Can you work these out from the model? Positions are in its coordinate system, mm. Face numbers are marked on the shaded views. A direction names the side the tool comes from. Round coordinates to 2 decimals unless told otherwise and drop trailing zeros. Loops run counter-clockwise (first coordinate to the right, second up) from the corner with the lowest first, then second, coordinate; pieces in that order, holes last.
(1) If I drill on line 1 along Y through (x, z) = (9.25, 10.5); line 2 along Z through (x, y) = (6.75, 50); line 3 along Y through (x, z) = (8.75, 5), over which ranges is the centre line in solid material (lowest first)?
(2) I want a section at B-B on x = 0. Write out the boundary of the cut face in (y, z), plus the area to 3 significant figures.
(3) Which directions (+Z, -Z, +X, -X, +Y, -Y) give clear straight access to the entire face, cutting with the end or side of a thin tool? Please do the marked faces 1, 2 and 3.
(4) I want a section at A-A on z = 8.5. Write out the boundary of the cut face in (x, y), plus the area to 3 significant figures.
(5) I want a section at C-C on x = -10.5. Write out the boundary of the cut face in (y, z), plus the area to 3 significant figures.
(6) Will these pins go through, and if not, where does the flat tip stop? pin 1 Ø14.5 at (x, y) = (1.5, 42.5) entering from +Z; pin 2 Ø5.5 at (x, y) = (1, 46.5) entering from -Z; pin 3 Ø6 at (y, z) = (-43, 12.5) entering from +X; pin 4 Ø9 at (y, z) = (53.5, 11) entering from -X.
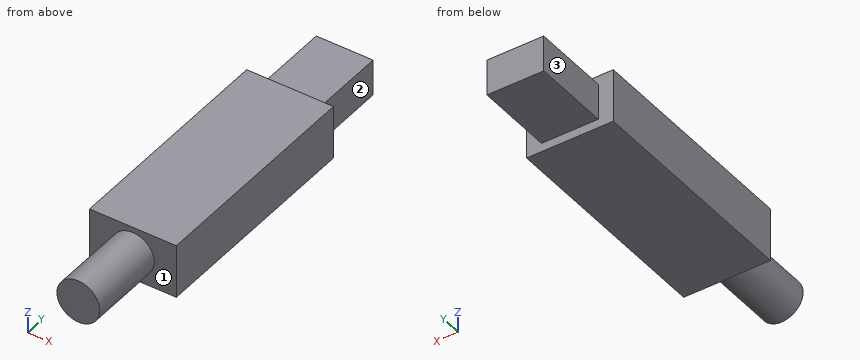
from build123d import *

# Parameters (mm, degrees)
F0_W     = 27.5
F0_H     = 72
F1_DEPTH = 17
F2_W     = 18
F2_H     = 11.5
F3_DEPTH = 25
F4_R     = 6.8
F5_DEPTH = 25


with BuildPart() as f1:
    # F0 (on Top) → F1 (new body)
    with BuildSketch(Plane.XY):
        Rectangle(F0_W, F0_H)
    extrude(amount=F1_DEPTH)

    # F2 (on face) → F3 (join)
    with BuildSketch(Plane(origin=(0, 36, 0), x_dir=(-1, 0, 0), z_dir=(0, 1, 0))):
        with Locations((0, 8.5)):
            Rectangle(F2_W, F2_H)
    extrude(amount=F3_DEPTH)

    # F4 (on face) → F5 (join)
    with BuildSketch(Plane.XZ.offset(36)):
        with Locations((0, 8.5)):
            Circle(F4_R)
    extrude(amount=F5_DEPTH)


solid = f1.part
Filled sheet:
1. line 1: y = -36 to 36
1. line 2: z = 2.75 to 14.25
1. line 3: y = -36 to 61
2. outline: (-61, 1.7) - (-36, 1.7) - (-36, 0) - (36, 0) - (36, 2.75) - (61, 2.75) - (61, 14.25) - (36, 14.25) - (36, 17) - (-36, 17) - (-36, 15.3) - (-61, 15.3) - close
2. area: 1,850 mm2
3. face 1: -Y
3. face 2: +Z, -Z, +X, +Y
3. face 3: +Z, -Z, -X, +Y
4. outline: (-13.75, -36) - (-6.8, -36) - (-6.8, -61) - (6.8, -61) - (6.8, -36) - (13.75, -36) - (13.75, 36) - (9, 36) - (9, 61) - (-9, 61) - (-9, 36) - (-13.75, 36) - close
4. area: 2,770 mm2
5. outline: (-36, 0) - (36, 0) - (36, 17) - (-36, 17) - close
5. area: 1,220 mm2
6. pin 1: stops at z = 17
6. pin 2: stops at z = 2.75
6. pin 3: stops at x = 6.73
6. pin 4: stops at x = -9
